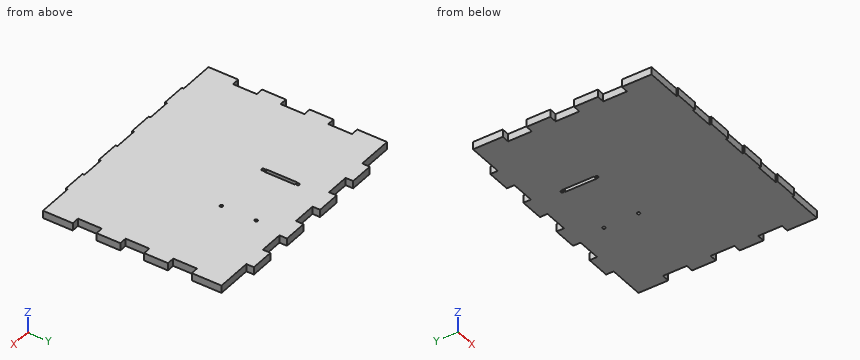
from build123d import *

# Parameters (mm, degrees)
SKETCH1_R           = 1.25
SKETCH1_W           = 3
SKETCH1_H           = 26.2
BOSS_EXTRUDE4_DEPTH = 6.35


with BuildPart() as part:
    # Sketch1 → Boss-Extrude4 (new body)
    with BuildSketch(Plane.XY):
        Polygon((0, 25), (0, 0), (30, 0), (30, -1.5875), (50, -1.5875), (50, 0), (70, 0), (70, -1.5875), (90, -1.5875), (90, 0), (110, 0), (110, -1.5875), (130, -1.5875), (130, 0), (150, 0), (150, -1.5875), (170, -1.5875), (170, 0), (200, 0), (200, 25), (193.65, 25), (193.65, 45), (200, 45), (200, 65), (193.65, 65), (193.65, 85), (200, 85), (200, 105), (193.65, 105), (193.65, 125), (200, 125), (200, 150), (170, 150), (170, 156.35), (150, 156.35), (150, 150), (130, 150), (130, 156.35), (110, 156.35), (110, 150), (90, 150), (90, 156.35), (70, 156.35), (70, 150), (50, 150), (50, 156.35), (30, 156.35), (30, 150), (0, 150), (0, 125), (6.35, 125), (6.35, 105), (0, 105), (0, 85), (6.35, 85), (6.35, 65), (0, 65), (0, 45), (6.35, 45), (6.35, 25), align=None)
        with Locations((74.769797365, 97.95)):
            Circle(SKETCH1_R, mode=Mode.SUBTRACT)
        with Locations((74.769797365, 112.5)):
            Rectangle(SKETCH1_W, SKETCH1_H, mode=Mode.SUBTRACT)
        with Locations((74.769797365, 127.05)):
            Circle(SKETCH1_R, mode=Mode.SUBTRACT)
        with Locations((125.230202635, 97.95)):
            Circle(SKETCH1_R, mode=Mode.SUBTRACT)
        with Locations((125.230202635, 127.05)):
            Circle(SKETCH1_R, mode=Mode.SUBTRACT)
    extrude(amount=BOSS_EXTRUDE4_DEPTH)


solid = part.part
Work out the finished part from the listing and answer in its coordinate system (mm). Round coordinates to 2 decimals unless told otherwise and drop trailing zeros. Write each loop counter-clockwise with the first axis right and the second up, starting at its lowest first coordinate (ties: lowest second). Pieces come first, ordered by that corner, then holes. Notation, with made-up numbers: (-10, 55) -> (16, 55) arc R31 ccw to (16, 85) -> close; hole circle Ø10 at (60, 61). An arc over 180 degrees is marked (long way). Answer as CSV lines item,"result". Start each with the question number.
(1) Find the intervals of material crossed by probe 1 along X at (y, z) = (127.05, 3); probe 2 along Y at (x, z) = (182.5, 1.25); probe 3 along X at (y, z) = (117, 3.25), in increasing order.
(2) The part is cut by section A-A, the plane z = 1.5. Give the number of separate pieces and of enclosed holes in the cut face, then the cut area to 3 significant figures.
(3) Each of these flat-tipped pins is pushed along its axis until it touches: pin 1 (3 mm diameter, centred on x = 18.5, z = 3, fed in from -Y); pin 2 (1.9 mm diameter, centred on y = 154.5, z = 2.5, fed in from -X); pin 3 (3 mm diameter, centred on y = 110, z = 3.5, fed in from +X). Where does it stop, or does it pass through?
(4) The part is cut by section B-B, the plane y = 78.5. Give the vertices of the cut face in (x, z).
Output values:
1,probe 1,"x = 0 to 73.52, 76.02 to 123.98, 126.48 to 200"
1,probe 2,"y = 0 to 150"
1,probe 3,"x = 6.35 to 73.27, 76.27 to 193.65"
2,separate pieces,"1"
2,enclosed holes,"5"
2,area,"29,800 mm²"
3,pin 1,"stops at y = 0"
3,pin 2,"stops at x = 30"
3,pin 3,"stops at x = 193.65"
4,outline,"(6.35, 0) -> (193.65, 0) -> (193.65, 6.35) -> (6.35, 6.35) -> close"
